from build123d import *

# Parameters (mm, degrees)
BOSS_EXTRUDE1_DEPTH = 350
SKETCH2_W           = 350
SKETCH2_H           = 22
BOSS_EXTRUDE2_DEPTH = 20


with BuildPart() as part:
    # Sketch1 → Boss-Extrude1 (new body)
    with BuildSketch(Plane.XY):
        Polygon((0, 0), (412, 0), (412, 149.9557), align=None)
    extrude(amount=BOSS_EXTRUDE1_DEPTH)

    # Sketch2 → Boss-Extrude2 (add)
    with BuildSketch(Plane(origin=(412, 0, 0), x_dir=(0, 0, -1), z_dir=(1, 0, 0))):
        with Locations((-175, 118.9557)):
            Rectangle(SKETCH2_W, SKETCH2_H)
    extrude(amount=BOSS_EXTRUDE2_DEPTH)


solid = part.part
The model under review builds one solid part; all positions refer to its coordinate system, in mm. A direction names the side the tool comes from. Coordinates: 2 decimals unless noted, no trailing zeros. Write each loop counter-clockwise with the first axis right and the second up, starting at its lowest first coordinate (ties: lowest second). Pieces come first, ordered by that corner, then holes. Notation, with made-up numbers: M -14,15 L 37,15 A23 ccw 37,38 Z; hole C 89.25,26.5 d1. An arc over 180 degrees is marked long. Put each result on its own line as item: value.
1) Wall thickness on probe 1 along Y at (x, z) = (116, 73); probe 2 along Y at (x, z) = (162, 273): over which ranges is each line inside the solid? List them lowest first. Write a range as [from, to].
Computed:
probe 1: y = [0, 42.22]
probe 2: y = [0, 58.96]
2) For faces 1 (the flat face through (422, 107.956, 177)), 2 (the flat face through (412, 140, 173)), 3 (the flat face through (309, 59, 0)), list the 3-axis set-ups (+Z, -Z, +X, -X, +Y, -Y) from which the entire face can be reached by the end or side of a thin tool; tool diameter is ignored.
Computed:
face 1: +Z, -Z, +X, -Y
face 2: +Z, -Z, +X, +Y
face 3: -Z, +X, -X, +Y, -Y
3) Add section C-C on x = 262. Give the boundary of the cut face in (y, z), then the cut area to 3 significant figures.
Computed:
outline: M 0,0 L 95.36,0 L 95.36,350 L 0,350 Z
area: 33,400 mm2
4) Add section B-B on y = 30. Give the boundary of the cut face in (x, z), then the cut area to 3 significant figures.
Computed:
outline: M 82.42,0 L 412,0 L 412,350 L 82.42,350 Z
area: 115,000 mm2
5) Add section A-A on z = 201. Give the boundary of the cut face in (x, y).
Computed:
outline: M 0,0 L 412,0 L 412,107.96 L 432,107.96 L 432,129.96 L 412,129.96 L 412,149.96 Z
6) Clearance check with flat-ended pins moving along their axes: pin 1 Ø10 at (x, z) = (424.5, 186) entering from -Y; pin 2 Ø10 at (y, z) = (138.5, 98) entering from +X; pin 3 Ø6 at (x, z) = (419, 247.5) entering from +Y. State where each tip first meets the part, or that it passes through.
Computed:
pin 1: stops at y = 107.96
pin 2: stops at x = 412
pin 3: stops at y = 129.96
